Could you check a few things on this model? Use its own coordinates, in mm. Face numbers are marked on the shaded views. Give positions to 0.01 mm unless a question says otherwise; leave off trailing zeros. Order: outer loops, then holes, each group sorted by start corner. A loop starts at its lowest first (then second) coordinate and runs counter-clockwise, first axis right, second up. Notation, with made-up numbers: (-34, 14) - (-14, 14) arc R14 ccw to (-14, 27) - close; hole circle Ø7 at (16.25, 47). An arc over 180 degrees is marked (long way). One line per question, with ' | ' between items. Start each with the question number.
1. I need wall thicknesses on probe 1 along X at (y, z) = (0.8, 6); probe 2 along X at (y, z) = (5.75, 17.5); probe 3 along Z at (x, y) = (-1.5, 0.75). Which ranges of each line are inside material? Lowest first, please. Write a range as from..to.
2. Imagine slicing it at B-B (z = 6). Please give me the cut outline in (x, y), and give its area (3 significant figures).
3. Imagine slicing it at A-A (y = 6). Please give me the cut outline in (x, z).
4. If we mould it in two halves opening along X, with no side actions, what happens to the marked faces 1, 2, 3 and 4? For each: released by +X, released by -X, zero draft, split by the parting line, or undercut.
5. Imagine slicing it at C-C (x = -1). Please give me the cut outline in (y, z).
6. Imagine slicing it at D-D (z = 2.5). Please give me the cut outline in (x, y).
7. For P1, Ø3, axis at x = 5, z = 19.5, coming from the +Y side; P2, Ø2.5, axis at x = -1, z = 21, coming from the +Y side; P3, Ø6, axis at x = 5.5, z = 7.5, coming from the +Y side, each with a flat end and sliding along its axis, tell me the tip position at first contact or that it passes through.
```python
from build123d import *

# Parameters (mm, degrees)
EXTRUDE_641_DEPTH   = 27
SKETCH_3_R          = 1.5
CUT_EXTRUDE_1_DEPTH = 29.964806231


with BuildPart() as part:
    # Sketch 298 → Extrude 641 (new body)
    with BuildSketch(Plane.XY):
        Polygon((-7.6, 1), (-7.6, 7), (-8.6, 7), (-8.6, 0), (8.6, 0), (8.6, 7), (7.6, 7), (7.6, 1), align=None)
    extrude(amount=EXTRUDE_641_DEPTH)

    # Sketch 3 → Cut-Extrude 1 (cut, through all)
    with BuildSketch(Plane(origin=(0, 1, 0), x_dir=(1, 0, 0), z_dir=(0, 1, 0))):
        with Locations(Location((-1, -6, 0), (0, 0, 270))):
            Circle(SKETCH_3_R)
        with Locations(Location((-1, -21, 0), (0, 0, 270))):
            Circle(SKETCH_3_R)
    extrude(amount=-CUT_EXTRUDE_1_DEPTH, mode=Mode.SUBTRACT)


solid = part.part
```
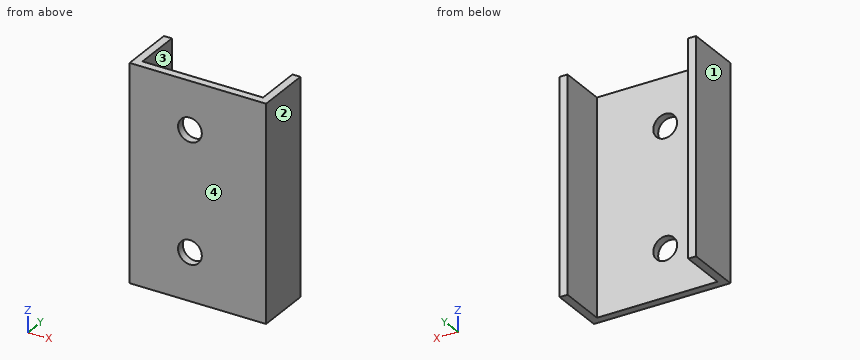
Results found:
1) probe 1: x = -8.6..-2.5, 0.5..8.6 | probe 2: x = -8.6..-7.6, 7.6..8.6 | probe 3: z = 0..4.59, 7.41..19.59, 22.41..27
2) outline: (-8.6, 0) - (-2.5, 0) - (-2.5, 1) - (-7.6, 1) - (-7.6, 7) - (-8.6, 7) - close; (0.5, 0) - (8.6, 0) - (8.6, 7) - (7.6, 7) - (7.6, 1) - (0.5, 1) - close | area: 26.2 mm2
3) outline: (-8.6, 0) - (-7.6, 0) - (-7.6, 27) - (-8.6, 27) - close; (7.6, 0) - (8.6, 0) - (8.6, 27) - (7.6, 27) - close
4) face 1: released by -X | face 2: released by +X | face 3: undercut | face 4: zero draft
5) outline: (0, 0) - (1, 0) - (1, 4.5) - (0, 4.5) - close; (0, 7.5) - (1, 7.5) - (1, 19.5) - (0, 19.5) - close; (0, 22.5) - (1, 22.5) - (1, 27) - (0, 27) - close
6) outline: (-8.6, 0) - (8.6, 0) - (8.6, 7) - (7.6, 7) - (7.6, 1) - (-7.6, 1) - (-7.6, 7) - (-8.6, 7) - close
7) P1: stops at y = 1 | P2: passes through | P3: stops at y = 7
